Part model, mm, in its own coordinate system. Face numbers are marked on the shaded views. A direction names the side the tool comes from. Give positions to 0.01 mm unless a question says otherwise; leave off trailing zeros. Write each loop counter-clockwise with the first axis right and the second up, starting at its lowest first coordinate (ties: lowest second). Pieces come first, ordered by that corner, then holes.
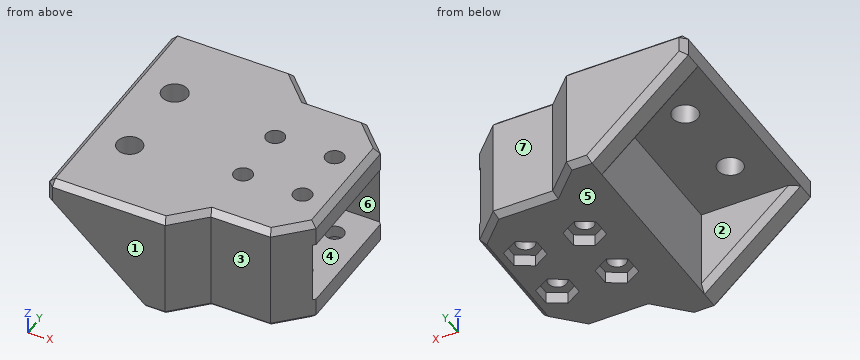
from build123d import *

# Parameters (mm, degrees)
SKETCH_1_W          = 40
SKETCH_1_H          = 30
SKETCH_1_R          = 2.15
SKETCH_1_R_2        = 2.1
SKETCH_1_R_3        = 1.55
EXTRUDE_1_DEPTH     = 4
CHAMFER_1_SIZE      = 5
EXTRUDE_2_DEPTH     = 10.4
EXTRUDE_START       = 4
SKETCH_4_R          = 1.55
EXTRUDE_3_DEPTH     = 4
EXTRUDE_4_DEPTH     = 5
EXTRUDE_5_DEPTH     = 5
CHAMFER_3_SIZE      = 10
CHAMFER_4_SIZE      = 1
CUT_EXTRUDE_1_DEPTH = 2
SKETCH_10_W         = 10.4
SKETCH_10_H         = 20.8
CUT_EXTRUDE_2_DEPTH = 43.806074335


with BuildPart() as part:
    # 草图1 → 凸台-拉伸1 (new body)
    with BuildSketch(Plane.XY):
        with Locations((20, 15)):
            Rectangle(SKETCH_1_W, SKETCH_1_H)
        with Locations((7, 22)):
            Circle(SKETCH_1_R, mode=Mode.SUBTRACT)
        with Locations((7, 8)):
            Circle(SKETCH_1_R_2, mode=Mode.SUBTRACT)
        with Locations((35, 20)):
            Circle(SKETCH_1_R_3, mode=Mode.SUBTRACT)
        with Locations((25, 20)):
            Circle(SKETCH_1_R_3, mode=Mode.SUBTRACT)
        with Locations((25, 10)):
            Circle(SKETCH_1_R_3, mode=Mode.SUBTRACT)
        with Locations((35, 10)):
            Circle(SKETCH_1_R_3, mode=Mode.SUBTRACT)
    extrude(amount=EXTRUDE_1_DEPTH)

    # 倒角1
    chamfer_1_edges = [part.edges().sort_by_distance(p)[0] for p in [
        (40, 30, 2),
        (40, 0, 2),
    ]]
    chamfer(chamfer_1_edges, length=CHAMFER_1_SIZE)

    # 草图3 → 凸台-拉伸2 (add)
    with BuildSketch(Plane(origin=(0, 0, 0), x_dir=(-1, 0, 0), z_dir=(0, 0, -1))):
        Polygon((-40, 25), (-20, 25), (-20, 5), (-40, 5), (-35, 0), (-16.2, 0), (-16.2, 30), (-35, 30), align=None)
    extrude(amount=EXTRUDE_2_DEPTH)

    # 草图4 → 凸台-拉伸3 (add)
    with BuildSketch(Plane(origin=(0, 0, -10.4), x_dir=(-1, 0, 0), z_dir=(0, 0, -1)).offset(EXTRUDE_START)):
        Polygon((-40, 25), (-40, 5), (-35, 0), (-16.2, 0), (-16.2, 30), (-35, 30), align=None)
        with Locations(Location((-35, 20, 0), (0, 0, 180))):
            Circle(SKETCH_4_R, mode=Mode.SUBTRACT)
        with Locations(Location((-25, 20, 0), (0, 0, 180))):
            Circle(SKETCH_4_R, mode=Mode.SUBTRACT)
        with Locations(Location((-25, 10, 0), (0, 0, 180))):
            Circle(SKETCH_4_R, mode=Mode.SUBTRACT)
        with Locations(Location((-35, 10, 0), (0, 0, 180))):
            Circle(SKETCH_4_R, mode=Mode.SUBTRACT)
    extrude(amount=-EXTRUDE_3_DEPTH)

    # 草图7 → 凸台-拉伸4 (add)
    with BuildSketch(Plane.XZ):
        Polygon((0, 0), (16.2, -14.4), (30, -14.4), (30, 4), (0, 4), align=None)
    extrude(amount=EXTRUDE_4_DEPTH)

    # 草图8 → 凸台-拉伸5 (add)
    with BuildSketch(Plane(origin=(0, 30, 0), x_dir=(1, 0, 0), z_dir=(0, 1, 0))):
        Polygon((0, 0), (16.2, 14.4), (30, 14.4), (30, -4), (0, -4), align=None)
    extrude(amount=EXTRUDE_5_DEPTH)

    # 倒角3
    # the kernel refuses this chamfer: 10 mm, written as the material it takes off along each edge
    with BuildSketch(Plane(origin=(30, 35, -40.11682988), x_dir=(-0.9996219169112968, 0.027495876610586317, 0), z_dir=(0, 0, 1))) as chamfer_3_piece_1_section:
        Polygon((CHAMFER_3_SIZE * 0.999621916911, CHAMFER_3_SIZE * 0.0274958766106), (-CHAMFER_3_SIZE * 0.0274958766106, CHAMFER_3_SIZE * 0.999621916911), (0, 0), align=None)
    chamfer_3_piece_1 = extrude(amount=69.833659759, mode=Mode.PRIVATE)
    chamfer_3_piece_1 = split(chamfer_3_piece_1, bisect_by=Plane(origin=(26.065989159, 30, -5.2), z_dir=(0, 1, 0)), keep=Keep.TOP, mode=Mode.PRIVATE)
    add(chamfer_3_piece_1, mode=Mode.SUBTRACT)
    with BuildSketch(Plane(origin=(30, -5, -40.11682988), x_dir=(-0.9996219169112968, -0.027495876610586403, 0), z_dir=(0, 0, 1))) as chamfer_3_piece_2_section:
        Polygon((CHAMFER_3_SIZE * 0.999621916911, -CHAMFER_3_SIZE * 0.0274958766106), (-CHAMFER_3_SIZE * 0.0274958766106, -CHAMFER_3_SIZE * 0.999621916911), (0, 0), align=None)
    chamfer_3_piece_2 = extrude(amount=69.833659759, mode=Mode.PRIVATE)
    chamfer_3_piece_2 = split(chamfer_3_piece_2, bisect_by=Plane(origin=(26.065989159, 0, -5.2), z_dir=(0, -1, 0)), keep=Keep.TOP, mode=Mode.PRIVATE)
    add(chamfer_3_piece_2, mode=Mode.SUBTRACT)

    # 倒角4
    chamfer_4_edges = [part.edges().sort_by_distance(p)[0] for p in [
        (30, 0, 4),
        (8.1, 0, -7.2),
        (0, -5, 2),
        (8.1, -5, -7.2),
        (18.1, -5, -14.4),
        (30, 30, -14.4),
        (8.1, 30, -7.2),
        (8.1, 35, -7.2),
        (0, 35, 2),
        (10, 35, 4),
        (18.1, 35, -14.4),
        (22.5, -2.5, -14.4),
        (22.5, 32.5, -14.4),
        (10, -5, 4),
        (22.5, -2.5, 4),
        (22.5, 32.5, 4),
        (40, 15, 4),
        (30, 30, 4),
        (37.5, 27.5, 4),
        (37.5, 2.5, 4),
        (0, 15, 4),
        (37.5, 27.5, -14.4),
        (40, 15, -14.4),
        (37.5, 2.5, -14.4),
        (30, 0, -14.4),
    ]]
    chamfer(chamfer_4_edges, length=CHAMFER_4_SIZE)

    # 草图9 → 切除-拉伸1 (cut)
    with BuildSketch(Plane(origin=(0, 0, -14.4), x_dir=(-1, 0, 0), z_dir=(0, 0, -1))):
        Polygon((-35, 16.766838493), (-32.2, 18.383419246), (-32.2, 21.616580754), (-35, 23.233161507), (-37.8, 21.616580754), (-37.8, 18.383419246), align=None)
        Polygon((26.245937902, 18.719863705), (29.045937902, 20.336444458), (29.045937902, 23.569605966), (26.245937902, 25.186186719), (23.445937902, 23.569605966), (23.445937902, 20.336444458), align=None)
        Polygon((-35, 6.766838493), (-32.2, 8.383419246), (-32.2, 11.616580754), (-35, 13.233161507), (-37.8, 11.616580754), (-37.8, 8.383419246), align=None)
        Polygon((-25, 6.766838493), (-22.2, 8.383419246), (-22.2, 11.616580754), (-25, 13.233161507), (-27.8, 11.616580754), (-27.8, 8.383419246), align=None)
        Polygon((-25, 16.766838493), (-22.2, 18.383419246), (-22.2, 21.616580754), (-25, 23.233161507), (-27.8, 21.616580754), (-27.8, 18.383419246), align=None)
    extrude(amount=-CUT_EXTRUDE_1_DEPTH, mode=Mode.SUBTRACT)

    # 草图10 → 切除-拉伸2 (cut, through all)
    with BuildSketch(Plane(origin=(20, 0, 0), x_dir=(0, 0, -1), z_dir=(1, 0, 0))):
        with Locations((5.2, 15)):
            Rectangle(SKETCH_10_W, SKETCH_10_H)
    extrude(amount=CUT_EXTRUDE_2_DEPTH, mode=Mode.SUBTRACT)


solid = part.part
1) Saw through at B-B (x = 6.5). Write the cut outline in (y, z), and give its area (3 significant figures).
Check result:
outline: (-5, -4.44) - (-4, -5.78) - (-1, -5.78) - (0, -4.44) - (0, 0) - (5.96, 0) - (5.96, 4) - (-4, 4) - (-5, 3) - close; (10.04, 0) - (19.91, 0) - (19.91, 4) - (10.04, 4) - close; (24.09, 0) - (30, 0) - (30, -4.44) - (31, -5.78) - (34, -5.78) - (35, -4.44) - (35, 3) - (34, 4) - (24.09, 4) - close
area: 181 mm2
2) Saw through at D-D (y = 1.5). Write the cut outline in (x, z).
Check result:
outline: (0, 0) - (16.2, 0) - (16.2, -14.4) - (35.09, -14.4) - (36.5, -13.4) - (36.5, 3) - (35.09, 4) - (1, 4) - (0, 3) - close
3) 3-axis set-ups, long thin cutter, end or side, ignore diameter. For the marked faces 1, 2 and 3: which of +Z, -Z, +X, -X, +Y, -Y reach the whole face in a straight line?
Check result:
face 1: +Z, -Z, +X, -X, -Y
face 2: -Z, -X
face 3: +Z, -Z, +X, -Y
4) Drill centre lines: L1, parallel to X at y = 20, z = -11.65; L2, parallel to Y at x = 35, z = 1.55; L3, parallel to X at y = 21, z = 2. Where is each one in solid material? Low to high.
Check result:
L1: x = 16.2 to 23.45, 26.55 to 33.45, 36.55 to 40
L2: y = 0 to 8.45, 11.55 to 18.45, 21.55 to 30
L3: x = 0 to 5.1, 8.9 to 23.82, 26.18 to 33.82, 36.18 to 40
5) Saw through at C-C (z = -11.75). Write the cut outline in (x, y).
Check result:
outline: (13.22, -4) - (14.72, -5) - (20, -5) - (25, 0) - (35, 0) - (40, 5) - (40, 25) - (35, 30) - (25, 30) - (20, 35) - (14.72, 35) - (13.22, 34) - (13.22, 31) - (14.72, 30) - (16.2, 30) - (16.2, 0) - (14.72, 0) - (13.22, -1) - close; hole circle Ø3.1 at (25, 10); hole circle Ø3.1 at (25, 20); hole circle Ø3.1 at (35, 10); hole circle Ø3.1 at (35, 20)
6) Flat gauge pins, fed straight in: P1, Ø4, axis at x = 35, y = 10, coming from the -Z side; P2, Ø1.9, axis at x = 35, y = 20, coming from the -Z side; P3, Ø2, axis at x = 29.5, z = -12, coming from the -Y side; P4, Ø5, axis at y = 29, z = -5.5, coming from the +X side. Where does each tip first touch, or does it go through?
Check result:
P1: stops at z = -12.4
P2: passes through
P3: stops at y = 0
P4: stops at x = 38.5
7) Mould opens along Z. For the marked faces 4, 5, 6 and 7 say: +Z half, -Z half, draft (parallel to the pull), parting line (faces both ways), or undercut.
Check result:
face 4: undercut
face 5: -Z half
face 6: undercut
face 7: draft
8) Saw through at A-A (z = 1.5). Write the cut outline in (x, y), and give its area (3 significant figures).
Check result:
outline: (0, -4) - (1, -5) - (20, -5) - (25, 0) - (35, 0) - (40, 5) - (40, 25) - (35, 30) - (25, 30) - (20, 35) - (1, 35) - (0, 34) - close; hole circle Ø4.3 at (7, 22); hole circle Ø4.2 at (7, 8); hole circle Ø3.1 at (25, 10); hole circle Ø3.1 at (25, 20); hole circle Ø3.1 at (35, 10); hole circle Ø3.1 at (35, 20)
area: 1,340 mm2
